Part model, mm, in its own coordinate system. Face numbers are marked on the shaded views. A direction names the side the tool comes from. Give positions to 0.01 mm unless a question says otherwise; leave off trailing zeros. Order: outer loops, then holes, each group sorted by start corner. A loop starts at its lowest first (then second) coordinate and runs counter-clockwise, first axis right, second up. Notation, with made-up numbers: (5.25, 32.5) - (23.25, 32.5) arc R14 ccw to (23.25, 44.5) - close; hole circle Ø8 at (-20.5, 64). An arc over 180 degrees is marked (long way). One line per item, written item: value.
```python
from build123d import *

# Parameters (mm, degrees)
SKETCH1_R               = 63.5
SKETCH1_R_2             = 152.4
BOSS_EXTRUDE1_DEPTH     = 127
CUT_EXTRUDE1_DEPTH      = 1264.634045125
CUT_EXTRUDE1_DEPTH_BACK = 1264.634045125
SKETCH2_W               = 101.6
SKETCH2_H               = 355.6
CUT_EXTRUDE2_DEPTH      = 254


with BuildPart() as part:
    # Sketch1 → Boss-Extrude1 (new, symmetric)
    with BuildSketch(Plane.XY):
        with BuildLine():
            Line((127, -294.794488402), (127, -762))
            ThreePointArc((127, -762), (0, -889), (-127, -762))
            Line((-127, -762), (-127, -508))
            ThreePointArc((-127, -508), (-238.592316368, -238.592316368), (-508, -127))
            Line((-508, -127), (-762, -127))
            ThreePointArc((-762, -127), (-889, 0), (-762, 127))
            Line((-762, 127), (-508, 127))
            ThreePointArc((-508, 127), (-238.592316368, 238.592316368), (-127, 508))
            Line((-127, 508), (-127, 762))
            ThreePointArc((-127, 762), (0, 889), (127, 762))
            Line((127, 762), (127.177644281, 294.893747175))
            ThreePointArc((127.177644281, 294.893747175), (139.582882613, 234.726570772), (174.736020462, 184.345662149))
            ThreePointArc((174.736020462, 184.345662149), (253.999988445, -0.076613885), (174.624780504, -184.451039666))
            ThreePointArc((174.624780504, -184.451039666), (139.476090274, -234.729960661), (127, -294.794488402))
        make_face()
        with Locations((0, 762)):
            Circle(SKETCH1_R, mode=Mode.SUBTRACT)
        with Locations((0, -762)):
            Circle(SKETCH1_R, mode=Mode.SUBTRACT)
        with Locations((-762, 0)):
            Circle(SKETCH1_R, mode=Mode.SUBTRACT)
        Circle(SKETCH1_R_2, mode=Mode.SUBTRACT)
    extrude(amount=BOSS_EXTRUDE1_DEPTH, both=True)

    # Sketch2 → Cut-Extrude1 (cut, two sides: drawn at the far end of the back side and taken through both)
    with BuildSketch(Plane(origin=(0, 0, 0), x_dir=(0, 0, -1), z_dir=(1, 0, 0)).offset(-CUT_EXTRUDE1_DEPTH_BACK)):
        Polygon((-50.8, 889), (50.8, 889), (50.8, 533.4), (0, 533.4), (-50.8, 533.4), align=None)
        with Locations((0, -711.2)):
            Rectangle(SKETCH2_W, SKETCH2_H)
    extrude(amount=CUT_EXTRUDE1_DEPTH + CUT_EXTRUDE1_DEPTH_BACK, mode=Mode.SUBTRACT)

    # Sketch3 → Cut-Extrude2 (cut)
    with BuildSketch(Plane(origin=(0, 127, 0), x_dir=(1, 0, 0), z_dir=(0, 1, 0))):
        with BuildLine():
            Line((-762, 127), (-762, 63.5))
            Line((-762, 63.5), (-596.9, 63.5))
            ThreePointArc((-596.9, 63.5), (-551.998719395, 82.098719395), (-533.4, 127))
            Line((-533.4, 127), (-762, 127))
        make_face()
        Polygon((-889, 63.5), (-762, 63.5), (-762, 127), (-533.4, 127), (-533.4, 247.034120233), (-889, 247.034120233), align=None)
        Polygon((-762, -127), (-762, -63.5), (-889, -63.5), (-889, -178.364595134), (-533.4, -178.364595134), (-533.4, -127), align=None)
        with BuildLine():
            ThreePointArc((-533.4, -127), (-551.998719395, -82.098719395), (-596.9, -63.5))
            Line((-596.9, -63.5), (-762, -63.5))
            Line((-762, -63.5), (-762, -127))
            Line((-762, -127), (-533.4, -127))
        make_face()
    extrude(amount=-CUT_EXTRUDE2_DEPTH, mode=Mode.SUBTRACT)


solid = part.part
```
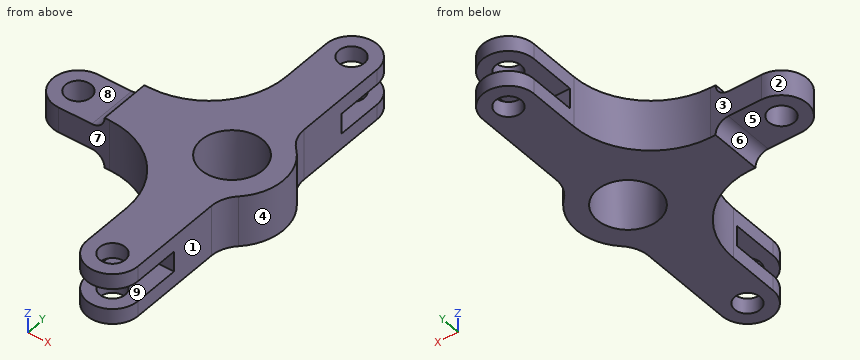
1) Mould opens along Z. For the marked faces 6, 7, 8 and 9 say: released by +Z, released by -Z, zero draft, split by the parting line, or undercut.
Outcome:
face 6: released by -Z
face 7: zero draft
face 8: released by +Z
face 9: undercut
2) Cut at A-A, the plane y = 0. Give the cut face in (x, z), then the cut area to 3 significant figures.
Outcome:
outline: (-889, -63.5) - (-825.5, -63.5) - (-825.5, 63.5) - (-889, 63.5) - close; (-698.5, -63.5) - (-596.9, -63.5) arc R63.5 cw to (-533.4, -127) - (-152.4, -127) - (-152.4, 127) - (-533.4, 127) arc R63.5 cw to (-596.9, 63.5) - (-698.5, 63.5) - close; (152.4, -127) - (254, -127) - (254, 127) - (152.4, 127) - close
area: 153,000 mm^2
3) Cut at C-C, the plane x = 0. Give the number of separate pieces and of enclosed holes in the cut face, then the cut area to 3 significant figures.
Outcome:
separate pieces: 6
enclosed holes: 0
area: 263,000 mm^2
4) Which spindle directions (+Z, -Z, +X, -X, +Y, -Y) get a long thin tool onto all of the face, cutting with end or side? Do the marked faces 1, 2, 3, 4 and 5. Say none if no direction does.
Outcome:
face 1: +Z, -Z, +X, -Y
face 2: +Z, -Z, -X
face 3: +Z, -Z, -X, +Y
face 4: +Z, -Z, +X
face 5: -Z, -X, +Y, -Y
5) Cut at B-B, the plane z = 33. Give the cut face in (x, y), then the cut area to 3 significant figures.
Outcome:
outline: (-762, -127) - (-508, -127) arc R381 cw to (-127, -508) - (-127, -533.4) - (127, -533.4) - (127, -294.79) arc R152.4 cw to (174.62, -184.45) arc R254 ccw to (174.74, 184.35) arc R152.4 cw to (127.18, 294.89) - (127.09, 533.4) - (-127, 533.4) - (-127, 508) arc R381 cw to (-508, 127) - (-762, 127) arc R127 ccw to start; hole circle Ø127 at (-762, 0); hole circle Ø304.8 at (0, 0)
area: 475,000 mm^2
6) Cut at D-D, the plane y = -730.5. Give the cut face in (x, z), then the cut area to 3 significant figures.
Outcome:
outline: (-127, -127) - (-55.14, -127) - (-55.14, -50.8) - (-127, -50.8) - close; (-127, 50.8) - (-55.14, 50.8) - (-55.14, 127) - (-127, 127) - close; (55.14, -127) - (127, -127) - (127, -50.8) - (55.14, -50.8) - close; (55.14, 50.8) - (127, 50.8) - (127, 127) - (55.14, 127) - close
area: 21,900 mm^2
7) Pin check, flat tips, straight feed: pin 1 (8 mm diameter, centred on y = -496.5, z = -99, fed in from +X); pin 2 (10 mm diameter, centred on x = -214.5, z = 67.5, fed in from +Y); pin 3 (10 mm diameter, centred on x = -550.5, z = 34, fed in from +Y). Stop position of each tip, or through.
Outcome:
pin 1: stops at x = 127
pin 2: stops at y = 271.23
pin 3: stops at y = 127
8) Drill centre lines: line 1 along Y through (x, z) = (0, 107.5); line 2 along X through (y, z) = (762, -93); line 3 along Z through (x, y) = (51, -811.5). Where is each one in solid material? Low to high. Write a range as from..to.
Outcome:
line 1: y = -889..-825.5, -698.5..-152.4, 152.4..698.5, 825.5..889
line 2: x = -127..-63.5, 63.5..127
line 3: z = -127..-50.8, 50.8..127
